The model under review builds one solid part; all positions refer to its coordinate system, in mm. Round coordinates to 2 decimals unless told otherwise and drop trailing zeros. Order: outer loops, then holes, each group sorted by start corner. A loop starts at its lowest first (then second) coordinate and runs counter-clockwise, first axis right, second up.
1) Consider section A-A (y = 20.8). Give the boundary of the cut face in (x, z), then the cut area to 3 significant figures.
2) Mouldability with a two-part tool opening along Y and no side actions: class faces 1 (the face through (0, 102, 49.8)), 2 (the face through (-19.846, 37.434, 50.54)) as pulls with the +Y half, pulls with the -Y half, needs draft (parallel to the pull), parting line crosses it, or undercut.
3) To check wall thickness, follow L1, parallel to X at y = 179.2, z = 50.5; L2, parallel to X at y = 77.5, z = 50.8; L3, parallel to Y at x = -1.5, z = 50.55. State the ranges of each line that lie inside material, in increasing order.
4) Clearance check with a flat-ended pin moving along its axis: P1, Ø3.5, axis at x = -14.4, y = 179.2, coming from the -Z side. State where the tip first meets the part, or that it passes through.
5) Consider section B-B (x = -20.8). Give the number of separate pieces and of enclosed holes in the cut face, then the cut area to 3 significant figures.
Autodesk Inventor part; units mm, degrees
ref_plane "Work Plane1" through (-24.15, -24.15, 49.8) normal (0, 0, 1) x (1, 0, 0)
ref_plane "YZ Plane" through (0, 0, 0) normal (1, 0, 0) x (0, 1, 0)
ref_plane "XZ Plane" through (0, 0, 0) normal (0, 1, 0) x (-1, 0, 0)
sketch "Sketch1" plane through (0, 0, 0) normal (0, 0, 1) x (1, 0, 0)
  circle A0 centre (-21.9, -21.9) radius 1.875
  circle A1 centre (21.9, 21.9) radius 1.875
  circle A2 centre (21.9, -21.9) radius 1.875
  circle A3 centre (-21.9, 21.9) radius 1.875
  circle A4 centre (14.4, 20.8) radius 2.0675
  circle A5 centre (-14.4, -20.8) radius 2.0675
  circle A6 centre (14.4, -20.8) radius 2.0675
  circle A7 centre (20.8, -14.4) radius 2.0675
  line L0 (-17.05, 17.05) -> (-17.05, -17.05)
  line L1 (17.05, 17.05) -> (-17.05, 17.05)
  line L2 (17.05, -17.05) -> (17.05, 17.05)
  line L3 (-17.05, -17.05) -> (17.05, -17.05)
  circle A8 centre (20.8, 14.4) radius 2.0675
  circle A9 centre (-14.4, 20.8) radius 2.0675
  circle A10 centre (-20.8, -14.4) radius 2.0675
  circle A11 centre (-20.8, 14.4) radius 2.0675
  line L4 (-22.9, 24.15) -> (22.9, 24.15)
  arc A12 (-22.9, 24.15) -> (-24.15, 22.9) centre (-22.9, 22.9) ccw
  line L5 (-24.15, -22.9) -> (-24.15, 22.9)
  arc A13 (-24.15, -22.9) -> (-22.9, -24.15) centre (-22.9, -22.9) ccw
  line L6 (22.9, -24.15) -> (-22.9, -24.15)
  arc A14 (22.9, -24.15) -> (24.15, -22.9) centre (22.9, -22.9) ccw
  line L7 (24.15, 22.9) -> (24.15, -22.9)
  arc A15 (24.15, 22.9) -> (22.9, 24.15) centre (22.9, 22.9) ccw
  point P0 (0, 0)
ref_plane "Work Plane1" through (-24.15, -24.15, 49.8) normal (0, 0, 1) x (1, 0, 0)
extrude "Extrusion1" add sketch "Sketch1" along normal blind 1.5 from surface at 49.8 contours A0 | A1 | A2 | A3 | L1 L2 L3 L0 | L4 A15 L7 A14 L6 A13 L5 A12
sketch "Sketch2" plane through (-22.9, -24.15, 51.3) normal (0, 0, 1) x (1, 0, 0)
  arc A0 (-1.25, 1.25) -> (0, 0) centre (0, 1.25) ccw
  line L0 (45.8, 0) -> (0, 0)
  arc A1 (45.8, 0) -> (47.05, 1.25) centre (45.8, 1.25) ccw
  line L1 (47.05, 47.05) -> (47.05, 1.25)
  arc A2 (47.05, 47.05) -> (45.8, 48.3) centre (45.8, 47.05) ccw
  line L2 (0, 48.3) -> (45.8, 48.3)
  arc A3 (0, 48.3) -> (-1.25, 47.05) centre (0, 47.05) ccw
  line L3 (-1.25, 1.25) -> (-1.25, 47.05)
  circle A4 centre (2.1, 38.55) radius 2.0675
  circle A5 centre (2.1, 9.75) radius 2.0675
  circle A6 centre (8.5, 44.95) radius 2.0675
  circle A7 centre (43.7, 38.55) radius 2.0675
  circle A8 centre (43.7, 9.75) radius 2.0675
  circle A9 centre (37.3, 3.35) radius 2.0675
  circle A10 centre (8.5, 3.35) radius 2.0675
  circle A11 centre (37.3, 44.95) radius 2.0675
  arc A12 (47.9, 47.05) -> (45.8, 49.15) centre (45.8, 47.05) ccw
  line L4 (47.9, 47.05) -> (47.9, 1.25)
  arc A13 (45.8, -0.85) -> (47.9, 1.25) centre (45.8, 1.25) ccw
  line L5 (45.8, -0.85) -> (0, -0.85)
  arc A14 (-2.1, 1.25) -> (0, -0.85) centre (0, 1.25) ccw
  line L6 (-2.1, 1.25) -> (-2.1, 47.05)
  arc A15 (0, 49.15) -> (-2.1, 47.05) centre (0, 47.05) ccw
  line L7 (0, 49.15) -> (45.8, 49.15)
  line L8 (47.05, 1.25) -> (45.8, 1.25)
  line L9 (45.8, 1.25) -> (45.8, -0.85)
  line L10 (45.8, -0.85) -> (47.05, -0.85)
  line L11 (47.05, -0.85) -> (47.05, 1.25)
  line L12 (-1.25, 1.25) -> (0, 1.25)
  line L13 (0, 1.25) -> (0, -0.85)
  line L14 (0, -0.85) -> (-1.25, -0.85)
  line L15 (-1.25, -0.85) -> (-1.25, 1.25)
  line L16 (-1.25, 47.05) -> (0, 47.05)
  line L17 (0, 47.05) -> (0, 49.15)
  line L18 (0, 49.15) -> (-1.25, 49.15)
  line L19 (-1.25, 49.15) -> (-1.25, 47.05)
  line L20 (47.05, 47.05) -> (45.8, 47.05)
  line L21 (45.8, 47.05) -> (45.8, 49.15)
  line L22 (45.8, 49.15) -> (47.05, 49.15)
  line L23 (47.05, 49.15) -> (47.05, 47.05)
  point P0 (22.9, 24.15)
  dimension "d2" = 0.85
extrude "Extrusion2" add sketch "Sketch2" against normal blind 1.5 contours A0 L13 A14 L15 | L0 L9 L5 L13 | L19 A15 L17 A3 | A14 L14 L15 | A1 L11 A13 L9 | L17 L7 L21 L2 | L19 L18 A15 | A13 L11 L10 | L21 A12 L23 A2 | L22 L23 A12
pattern_linear "Rectangular Pattern1" count 5 spacing 50 along (0, 1, 0) of "Extrusion1", "Extrusion2"
chamfer "Chamfer1" distance 1.5 angle 45 2 edges at (0, -25, 51.3) (0, 225, 51.3)
properties part number "Panel Top 1x5"
Answer below:
1. outline: (-24.15, 49.8) - (-16.47, 49.8) - (-16.47, 51.3) - (-24.15, 51.3) - close; (-12.33, 49.8) - (12.33, 49.8) - (12.33, 51.3) - (-12.33, 51.3) - close; (16.47, 49.8) - (24.15, 49.8) - (24.15, 51.3) - (16.47, 51.3) - close
1. area: 60.0 mm2
2. face 1: needs draft
2. face 2: undercut
3. L1: x = -24.15 to -16.47, -12.33 to 12.33, 16.47 to 24.15
3. L2: x = -24.15 to -15.58, -13.22 to 13.22, 15.58 to 24.15
3. L3: y = -24.25 to 224.25
4. P1: passes through
5. separate pieces: 11
5. enclosed holes: 0
5. area: 311 mm2
